```python
from build123d import *

# Parameters (mm, degrees)
F1_DEPTH = 50
F2_DEPTH = 100


with BuildPart() as f1:
    # F0 (on Top) → F1 (new body)
    with BuildSketch(Plane.XY):
        Polygon((-2.5, 5), (-20, 5), (-20, 0), (20, 0), (20, 5), (2.5, 5), align=None)
        with BuildLine():
            Line((-2.5, 20), (-2.5, 5))
            Line((-2.5, 5), (2.5, 5))
            Line((2.5, 5), (2.5, 20))
            ThreePointArc((2.5, 20), (0, 19.330127), (-2.5, 20))
        make_face()
        with BuildLine():
            ThreePointArc((5, 24.330127), (-2.5, 28.660254), (-2.5, 20))
            Line((-2.5, 20), (2.5, 20))
            ThreePointArc((2.5, 20), (4.330127, 21.830127), (5, 24.330127))
        make_face()
        with BuildLine():
            Line((2.5, 20), (-2.5, 20))
            ThreePointArc((-2.5, 20), (0, 19.330127), (2.5, 20))
        make_face()
    extrude(amount=F1_DEPTH)

    # F0 (on Top) → F2 (join)
    with BuildSketch(Plane.XY):
        with BuildLine():
            Line((2.5, 20), (-2.5, 20))
            ThreePointArc((-2.5, 20), (0, 19.330127), (2.5, 20))
        make_face()
        with BuildLine():
            ThreePointArc((5, 24.330127), (-2.5, 28.660254), (-2.5, 20))
            Line((-2.5, 20), (2.5, 20))
            ThreePointArc((2.5, 20), (4.330127, 21.830127), (5, 24.330127))
        make_face()
    extrude(amount=F2_DEPTH)


solid = f1.part
```
Geometry check sheet. Reference: the model listing, model coordinates, mm. A direction names the side the tool comes from. Round coordinates to 2 decimals unless told otherwise and drop trailing zeros. Order: outer loops, then holes, each group sorted by start corner. A loop starts at its lowest first (then second) coordinate and runs counter-clockwise, first axis right, second up. Notation, with made-up numbers: M 58.25,-38 L 79.25,-38 A17 cw 79.25,-33 Z; hole C 47.25,-23.5 d3. An arc over 180 degrees is marked long. Write item = value, one per line.
Q1. Release check for a two-part mould opening along Y. For faces 3 (the flat face through (-2.5, 13, 25)), 4 (the flat face through (-20, 3, 25)), 5 (the flat face through (0, 0, 25)) record: released by +Y, released by -Y, zero draft, split by the parting line, or undercut.
Answer block:
face_3 = undercut
face_4 = zero draft
face_5 = released by -Y
Q2. Section check B-B (y = 7). Enter the section's corners in (x, z), plus the area to 3 significant figures.
Answer block:
outline = M -2.5,0 L 2.5,0 L 2.5,50 L -2.5,50 Z
area = 250 mm^2
Q3. Set-up check for faces 1 (the flat face through (20, 2, 25)), 2 (the flat face through (2.5, 12, 25)): record each of +Z, -Z, +X, -X, +Y, -Y from which the full face is reachable in a straight line by a thin tool's end or side.
Answer block:
face_1 = +Z, -Z, +X, +Y, -Y
face_2 = +Z, -Z, +X
Q4. Scan lines: line 1 (X direction, y = 8.25, z = 7.5); line 2 (Z direction, x = -0.5, y = 4); line 3 (Y direction, x = -3.5, z = 6.5). Record each from-to range of solid material in increasing order.
Answer block:
line_1 = -2.5 to 2.5
line_2 = 0 to 50
line_3 = 0 to 5, 20.76 to 27.9
Q5. Section check C-C (z = 55). Enter the section's corners in (x, y).
Answer block:
outline = C 0,24.33 d10
Q6. Section check D-D (x = -12). Enter the section's corners in (y, z), plus the area to 3 significant figures.
Answer block:
outline = M 0,0 L 5,0 L 5,50 L 0,50 Z
area = 250 mm^2
Q7. Section check A-A (x = 0). Enter the section's corners in (y, z), plus the area to 3 significant figures.
Answer block:
outline = M 0,0 L 29.33,0 L 29.33,100 L 19.33,100 L 19.33,50 L 0,50 Z
area = 1,970 mm^2
Q8. Depth check by flat-ended pin: pin 1 Ø19 at (x, z) = (9.5, 29) entering from +Y; pin 2 Ø6 at (x, y) = (-5, 14) entering from +Z; pin 3 Ø6 at (x, y) = (-9, 9.5) entering from +Z; pin 4 Ø1 at (y, z) = (6, 13.5) entering from +X. Enter the tip coordinate at first touch or a pass-through.
Answer block:
pin_1 = 29.33
pin_2 = 50
pin_3 = through
pin_4 = 2.5
